from build123d import *

# Parameters (mm, degrees)
BOSS_EXTRUDE3_START      = -5
BOSS_EXTRUDE3_DEPTH      = 95
CUT_EXTRUDE1_DEPTH       = 211.669436796
CUT_EXTRUDE1_DEPTH_BACK  = 211.669436796
BOSS_EXTRUDE10_DEPTH     = 95
CUT_EXTRUDE2_DEPTH       = 211.669436796
CUT_EXTRUDE2_DEPTH_BACK  = 211.669436796
CUT_EXTRUDE7_DEPTH       = 211.669436796
CUT_EXTRUDE7_DEPTH_BACK  = 211.669436796
CUT_EXTRUDE12_START      = -3
CUT_EXTRUDE12_DEPTH      = 3
CUT_EXTRUDE18_DEPTH      = 263.682253196
CUT_EXTRUDE18_DEPTH_BACK = 263.682253196
CUT_EXTRUDE23_START      = -2
SKETCH26_W               = 5.160164367
SKETCH26_H               = 12.42
CUT_EXTRUDE23_DEPTH      = 207.011897718


# Read off the part's stored shape, not the designer's step: Cut-Extrude12
with BuildPart() as part:
    # Sketch4 → Boss-Extrude3 (new body)
    with BuildSketch(Plane(origin=(0, 0, 0), x_dir=(1, 0, 0), z_dir=(0, 1, 0)).offset(BOSS_EXTRUDE3_START)):
        Polygon((0, 54.04), (-30.96, 85), (170.46, 85), (139.5, 54.04), (139.5, 0), (0, 0), align=None)
    extrude(amount=BOSS_EXTRUDE3_DEPTH)

    # Sketch5 → Cut-Extrude1 (cut, two sides: drawn at the far end of the back side and taken through both)
    with BuildSketch(Plane(origin=(139.5, 0, 0), x_dir=(0, 0, -1), z_dir=(1, 0, 0)).offset(-CUT_EXTRUDE1_DEPTH_BACK)):
        Polygon((0, 90), (3, -3), (54.04, -2), (85, -5), (85, 90), align=None)
    extrude(amount=CUT_EXTRUDE1_DEPTH + CUT_EXTRUDE1_DEPTH_BACK, mode=Mode.SUBTRACT)

    # Sketch12 → Boss-Extrude10 (add)
    with BuildSketch(Plane.XZ.offset(5)):
        Polygon((77.75, 0), (61.75, 0), (5.136208879, -51.905643893), (1.313057643, -55.410852123), (-30.96, -85), (-26.520771025, -85), (62.809775082, -3.09840989), (69.75, -3), (76.690224918, -3.09840989), (166.020771025, -85), (170.46, -85), (138.186942357, -55.410852123), (134.363791121, -51.905643893), align=None)
    extrude(amount=-BOSS_EXTRUDE10_DEPTH)

    # Sketch6 → Cut-Extrude2 (cut, two sides: drawn at the far end of the back side and taken through both)
    with BuildSketch(Plane(origin=(139.5, 0, 0), x_dir=(0, 0, -1), z_dir=(1, 0, 0)).offset(-CUT_EXTRUDE2_DEPTH_BACK)):
        Polygon((54.04, 90), (0, 90), (54.04, 10.932684034), align=None)
    extrude(amount=CUT_EXTRUDE2_DEPTH + CUT_EXTRUDE2_DEPTH_BACK, mode=Mode.SUBTRACT)

    # Sketch18 → Cut-Extrude7 (cut, two sides: drawn at the far end of the back side and taken through both)
    with BuildSketch(Plane(origin=(0, 0, 0), x_dir=(1, 0, 0), z_dir=(0, 1, 0)).offset(-CUT_EXTRUDE7_DEPTH_BACK)):
        Polygon((-30.96, 85), (-32.039877687, 0), (5, 0), (5, 51.757080067), align=None)
        Polygon((61.75, 0), (5, 0), (5, 51.757080067), align=None)
        Polygon((134.5, 0), (77.75, 0), (134.5, 51.757080067), align=None)
        Polygon((170.46, 0), (134.5, 0), (134.5, 51.757080067), (170.46, 85), align=None)
    extrude(amount=CUT_EXTRUDE7_DEPTH + CUT_EXTRUDE7_DEPTH_BACK, mode=Mode.SUBTRACT)

    # Cut-Extrude12 outline → Cut-Extrude12 (cut)
    with BuildSketch(Plane(origin=(37.313647502, 0, 37.073562316), x_dir=(0.7370914330343759, 0, -0.6757930299635608), z_dir=(0.6757930299635608, 0, 0.7370914330343759)).offset(CUT_EXTRUDE12_START)):
        Polygon((134.824655296, 90), (134.824655296, 10.932684034), (180.637498322, -5), (180.637498322, 90), align=None)
    cut_extrude12 = extrude(amount=CUT_EXTRUDE12_DEPTH, mode=Mode.SUBTRACT)

    # Sketch24 → Cut-Extrude18 (cut, two sides: drawn at the far end of the back side and taken through both)
    with BuildSketch(Plane(origin=(-45.105018851, -43.594474596, -16.544137217), x_dir=(-6.841846231332114e-05, 0.3790169981348638, -0.9253897073361853), z_dir=(0.999999997266826, 0, -7.393475590237281e-05)).offset(-CUT_EXTRUDE18_DEPTH_BACK)):
        Polygon((55.352567213, 36.252396593), (85.320423961, 109.420477175), (87.366853148, 108.582309818), (57.398996399, 35.414229236), align=None)
    extrude(amount=CUT_EXTRUDE18_DEPTH + CUT_EXTRUDE18_DEPTH_BACK, mode=Mode.SUBTRACT)

    # Mirror4: Cut-Extrude12 across plane
    add(cut_extrude12.mirror(Plane(origin=(69.75, 0, 0), x_dir=(0, 0, 1), z_dir=(1, 0, 0))), mode=Mode.SUBTRACT)

    # Sketch26 → Cut-Extrude23 (cut)
    with BuildSketch(Plane(origin=(35.508131054, 0, 38.728927412), x_dir=(0.7370914330343759, 0, -0.6757930299635608), z_dir=(0.6757930299635608, 0, 0.7370914330343759)).offset(CUT_EXTRUDE23_START)):
        Polygon((67.688858918, 28.61), (85.688858918, 28.61), (92.688858918, 22.4), (85.688858918, 16.19), (67.688858918, 16.19), align=None)
        with Locations((54.728776735, 22.4)):
            Rectangle(SKETCH26_W, SKETCH26_H)
        Polygon((67.688858918, 16.19), (67.688858918, 28.61), (60.239227379, 28.61), (60.832079248, 16.19), align=None)
        Polygon((60.832079248, 16.19), (60.239227379, 28.61), (57.308858918, 28.61), (57.308858918, 16.19), align=None)
    cut_extrude23 = extrude(amount=CUT_EXTRUDE23_DEPTH, mode=Mode.SUBTRACT)

    # Mirror5: Cut-Extrude23 across plane
    add(cut_extrude23.mirror(Plane(origin=(69.75, 0, 0), x_dir=(0, 0, 1), z_dir=(1, 0, 0))), mode=Mode.SUBTRACT)


solid = part.part
Could you check a few things on this model? Use its own coordinates, in mm. A direction names the side the tool comes from. Round coordinates to 2 decimals unless told otherwise and drop trailing zeros. Write each loop counter-clockwise with the first axis right and the second up, starting at its lowest first coordinate (ties: lowest second). Pieces come first, ordered by that corner, then holes. Notation, with made-up numbers: (65.25, 31.5) - (113.25, 31.5) arc R14 ccw to (113.25, 35.5) - close; hole circle Ø1 at (-24.75, 30.25). An arc over 180 degrees is marked (long way). Use a Markdown table: item, result.
Q1. For faces 1 (the flat face through (38.901, 19.338, -22.325)), 2 (the flat face through (68.4, -3.48, -69.3)), 3 (the flat face through (49.6, 68.2, -14.9)), which set-ups out of +Z, -Z, +X, -X, +Y, -Y let a thin tool reach every point of the face, with its end or its side?
Output values:
| item | result |
|---|---|
| face 1 | +Z |
| face 2 | -Z, +Y |
| face 3 | -Z, +X, -X, +Y |
Q2. For pin 1 (16.5 mm diameter, centred on x = 89.5, z = -12.5, fed in from +Y); pin 2 (1 mm diameter, centred on x = 24, z = -50, fed in from +Y); pin 3 (16.5 mm diameter, centred on x = 53.5, z = -12.5, fed in from +Y); pin 4 (4 mm diameter, centred on x = 44.5, z = -11.5, fed in from -Y), each with a flat end and sliding along its axis, tell me the tip position at first contact or that it passes through.
Output values:
| item | result |
|---|---|
| pin 1 | y = 81.14 |
| pin 2 | y = -2.07 |
| pin 3 | y = 82.96 |
| pin 4 | through |
Q3. I want a section at B-B (z = -61.5). List the corners of the cut face in (x, y) for me.
Output values:
| item | result |
|---|---|
| outline | (-5.54, -5) - (145.04, -5) - (145.04, -2.72) - (144.83, -2.72) - (144.83, 7.09) - (140.39, 8.23) - (140.39, -2.72) - (-0.89, -2.72) - (-0.89, 8.23) - (-5.33, 7.09) - (-5.33, -2.72) - (-5.54, -2.72) - close |
Q4. Please list where these lines run through material, in increasing order: L1, parallel to Y at x = 123.5, z = -65; L2, parallel to X at y = 11, z = -21; L3, parallel to X at y = 7.5, z = -32.5.
Output values:
| item | result |
|---|---|
| L1 | -5 to -3.06 |
| L2 | 38.85 to 43.28, 96.22 to 100.65 |
| L3 | 26.3 to 30.74, 108.76 to 113.2 |
Q5. I want a section at C-C (x = 130). List the corners of the cut face in (y, z) for me.
Output values:
| item | result |
|---|---|
| outline | (-5, -85) - (-2, -54.04) - (-2.04, -51.97) - (13.95, -51.97) - (19.91, -47.9) - (-2.12, -47.9) - (-2.13, -47.65) - (-5, -47.65) - close |
